Geometry check sheet. Reference: drawing and pictorial views, mm from the part's lowest x, y, z. A direction names the side the tool comes from. Round coordinates to 2 decimals unless told otherwise and drop trailing zeros. Order: outer loops, then holes, each group sorted by start corner. A loop starts at its lowest first (then second) coordinate and runs counter-clockwise, first axis right, second up.
(1) Cross-section at B-B on y = 23.75. Enter the section's corners in (x, z) (1 decimal).
(2) Cross-section at A-A on x = 30. Enter the section's corners in (y, z).
(3) Thickness scan on L1, parallel to Z at x = 27, y = 5; L2, parallel to X at y = 23, z = 0.45; L3, parallel to X at y = 43.5, z = 0.7. Record the ranges inside material, lowest first.
(4) Cross-section at C-C on y = 42.5. Enter the section's corners in (x, z).
(5) Set-up check for the marked faces 1 and 2: record each of +Z, -Z, +X, -X, +Y, -Y from which the full face is reachable in a straight line by a thin tool's end or side.
(6) Cross-section at D-D on x = 7. Enter the section's corners in (y, z).
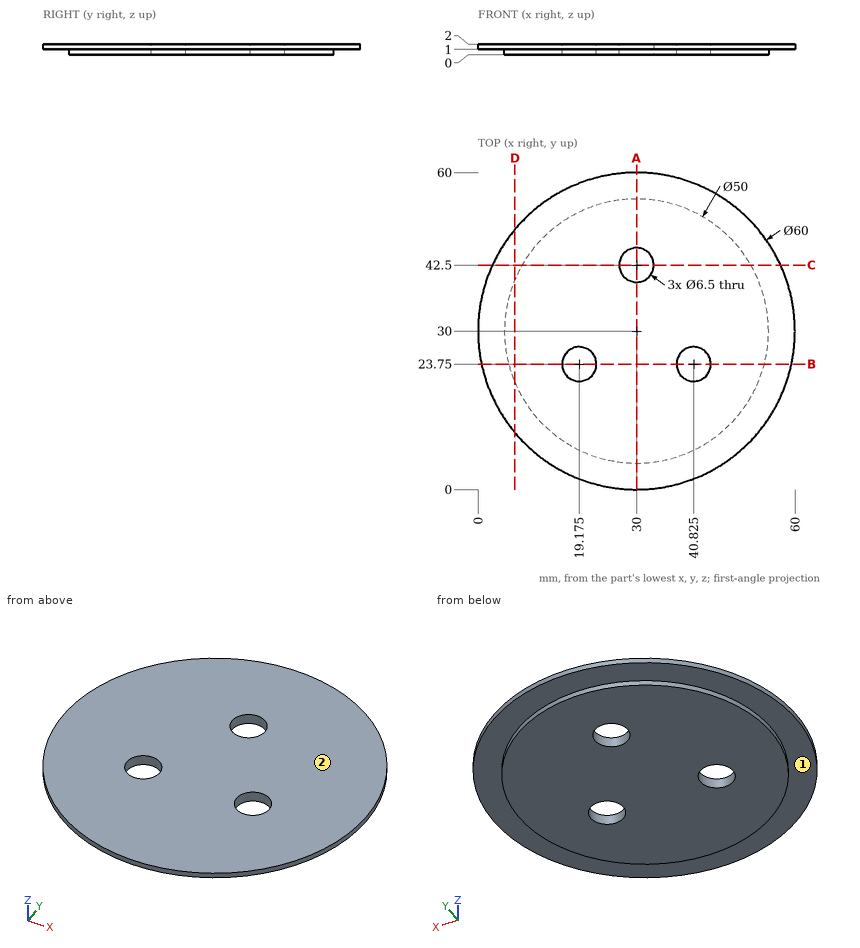
Found:
1. outline: (0.7, 1) - (5.8, 1) - (5.8, 0) - (15.9, 0) - (15.9, 2) - (0.7, 2) - close; (22.4, 0) - (37.6, 0) - (37.6, 2) - (22.4, 2) - close; (44.1, 0) - (54.2, 0) - (54.2, 1) - (59.3, 1) - (59.3, 2) - (44.1, 2) - close
2. outline: (0, 1) - (5, 1) - (5, 0) - (39.25, 0) - (39.25, 2) - (0, 2) - close; (45.75, 0) - (55, 0) - (55, 1) - (60, 1) - (60, 2) - (45.75, 2) - close
3. L1: z = 1 to 2
3. L2: x = 6 to 16.01, 22.34 to 37.66, 43.99 to 54
3. L3: x = 8.96 to 26.91, 33.09 to 51.04
4. outline: (2.73, 1) - (8.35, 1) - (8.35, 0) - (26.75, 0) - (26.75, 2) - (2.73, 2) - close; (33.25, 0) - (51.65, 0) - (51.65, 1) - (57.27, 1) - (57.27, 2) - (33.25, 2) - close
5. face 1: -Z
5. face 2: +Z, +X, -X, +Y, -Y
6. outline: (10.74, 1) - (20.2, 1) - (20.2, 0) - (39.8, 0) - (39.8, 1) - (49.26, 1) - (49.26, 2) - (10.74, 2) - close
